from build123d import *

# Parameters (mm, degrees)
SKETCH_1_W          = 9
SKETCH_1_H          = 9
EXTRUDE_1_DEPTH     = 235
SKETCH_2_W          = 7
SKETCH_2_H          = 7
CUT_EXTRUDE_1_DEPTH = 235
SKETCH_3_R          = 1.5
CUT_EXTRUDE_2_DEPTH = 235
CUT_EXTRUDE_3_DEPTH = 235
SKETCH_5_R          = 1.6
CUT_EXTRUDE_4_DEPTH = 10


with BuildPart() as part:
    # ｽｹｯﾁ1 → ﾎﾞｽ - 押し出し1 (new body)
    with BuildSketch(Plane.XY):
        Rectangle(SKETCH_1_W, SKETCH_1_H)
    extrude(amount=EXTRUDE_1_DEPTH)

    # ｽｹｯﾁ2 → ｶｯﾄ - 押し出し1 (cut)
    with BuildSketch(Plane.XY.offset(235)):
        Rectangle(SKETCH_2_W, SKETCH_2_H)
    extrude(amount=-CUT_EXTRUDE_1_DEPTH, mode=Mode.SUBTRACT)

    # ｽｹｯﾁ3 → ｶｯﾄ - 押し出し2 (cut)
    with BuildSketch(Plane(origin=(0, 4.5, 0), x_dir=(1, 0, 0), z_dir=(0, 1, 0))):
        with Locations((0, -5)):
            Circle(SKETCH_3_R)
        with Locations((0, -108)):
            Circle(SKETCH_3_R)
        with Locations((0, -225)):
            Circle(SKETCH_3_R)
    extrude(amount=-CUT_EXTRUDE_2_DEPTH, mode=Mode.SUBTRACT)

    # ｽｹｯﾁ4 → ｶｯﾄ - 押し出し3 (cut)
    with BuildSketch(Plane(origin=(0, 4.5, 0), x_dir=(1, 0, 0), z_dir=(0, 1, 0))):
        Polygon((4.5, -235), (-4.5, -235), (5.898758527, -230.150979263), align=None)
    extrude(amount=-CUT_EXTRUDE_3_DEPTH, mode=Mode.SUBTRACT)

    # ｽｹｯﾁ5 → ｶｯﾄ - 押し出し4 (cut)
    with BuildSketch(Plane(origin=(4.5, 0, 0), x_dir=(0, 0, -1), z_dir=(1, 0, 0))):
        with Locations((-221.153231077, 0)):
            Circle(SKETCH_5_R)
    extrude(amount=-CUT_EXTRUDE_4_DEPTH, mode=Mode.SUBTRACT)


solid = part.part
The model under review builds one solid part; all positions refer to its coordinate system, in mm. A direction names the side the tool comes from. Round coordinates to 2 decimals unless told otherwise and drop trailing zeros. Loops run counter-clockwise (first coordinate to the right, second up) from the corner with the lowest first, then second, coordinate; pieces in that order, holes last. Notation, with made-up numbers: (60, -25) -> (103, -25) arc R33 ccw to (103, 5) -> close; hole circle Ø3 at (39, -13). An arc over 180 degrees is marked (long way). Answer as CSV lines item,"result".
1) Add section B-B on x = 0. State how many separate pieces and enclosed holes the cut face has, plus the area to 3 significant figures.
Geometry results:
separate pieces,"8"
enclosed holes,"0"
area,"448 mm²"
2) Tool access review of faces 4 (the face through (3.5, 0, 117)), 5 (the face through (-0.06, -3.94, 232.93)): name each direction out of +Z, -Z, +X, -X, +Y, -Y from which nothing blocks a thin tool from reaching the whole face with its end or side.
Geometry results:
face 4,"+Z, -Z"
face 5,"+Z, +X, +Y, -Y"
3) Add section A-A on z = 145.5. Write out the cut boundary in (x, y).
Geometry results:
outline,"(-4.5, -4.5) -> (4.5, -4.5) -> (4.5, 4.5) -> (-4.5, 4.5) -> close; hole (-3.5, -3.5) -> (3.5, -3.5) -> (3.5, 3.5) -> (-3.5, 3.5) -> close"
4) To check wall thickness, follow line 1 along Y through (x, z) = (-2.75, 67); line 2 along X through (y, z) = (3.8, 225). State the ranges of each line that lie inside material, in increasing order. Write a range as from..to.
Geometry results:
line 1,"y = -4.5..-3.5, 3.5..4.5"
line 2,"x = -4.5..-1.5, 1.5..4.5"
5) Draft analysis for pull direction X (two halves, no side actions). For faces 1 (the face through (0, -4.5, 116)), 2 (the face through (0, -3.5, 119)), 3 (the face through (-4.5, 0, 116)), state which applies: pulls with the +X half, pulls with the -X half, needs draft (parallel to the pull), parting line crosses it, or undercut.
Geometry results:
face 1,"needs draft"
face 2,"undercut"
face 3,"pulls with the -X half"
